The listing builds one solid part. Answer for the finished solid, in the listing's coordinates (mm). A direction names the side the tool comes from. Coordinates: 2 decimals unless noted, no trailing zeros. Order: outer loops, then holes, each group sorted by start corner. A loop starts at its lowest first (then second) coordinate and runs counter-clockwise, first axis right, second up. Notation, with made-up numbers: (-38.5, 4) -> (-15.5, 4) arc R25 cw to (-15.5, 34) -> close; hole circle Ø11 at (11.25, 79). An arc over 180 degrees is marked (long way). Answer in a Markdown table with one row per item.
```python
from build123d import *

# Parameters (mm, degrees)
BOSS_EXTRUDE1_DEPTH     = 37.5
SHELL1_T                = -10
SKETCH2_W               = 230
SKETCH2_H               = 15
BOSS_EXTRUDE3_DEPTH     = 75
SKETCH1_4_OUTSIDE_W     = 306.9
SKETCH1_4_OUTSIDE_H     = 141.9
CUT_EXTRUDE2_DEPTH      = 38.5
CUT_EXTRUDE2_DEPTH_BACK = 38.5
SKETCH4_W               = 10
SKETCH4_H               = 75
SKETCH4_R               = 2.5
BOSS_EXTRUDE4_DEPTH     = 5
FILLET1_R               = 10
SKETCH3_R               = 3.75
CUT_EXTRUDE3_DEPTH      = 35
CUT_EXTRUDE4_START      = -75
SKETCH3_13_R            = 15
CUT_EXTRUDE4_DEPTH      = 35
CUT_EXTRUDE5_START      = -5
CUT_EXTRUDE5_DEPTH      = 65
CUT_EXTRUDE6_START      = -5
CUT_EXTRUDE6_DEPTH      = 30


with BuildPart() as part:
    # Sketch1 → Boss-Extrude1 (new body, symmetric)
    with BuildSketch(Plane.XY):
        with BuildLine():
            Line((125, 0), (-125, 0))
            Line((-125, 0), (-125, -15))
            ThreePointArc((-125, -15), (-104.497474683, -64.497474683), (-55, -85))
            Line((-55, -85), (45, -85))
            ThreePointArc((45, -85), (101.568542495, -61.568542495), (125, -5))
            Line((125, -5), (125, 0))
        make_face()
    extrude(amount=BOSS_EXTRUDE1_DEPTH, both=True)

    # Shell1
    shell1_openings = [part.faces().sort_by_distance(p)[0] for p in [
        (0, 0, 0),
    ]]
    offset(amount=SHELL1_T, openings=shell1_openings, kind=Kind.INTERSECTION)

    # Sketch2 → Boss-Extrude3 (add)
    with BuildSketch(Plane(origin=(0, 0, 0), x_dir=(1, 0, 0), z_dir=(0, 1, 0))):
        Rectangle(SKETCH2_W, SKETCH2_H)
    extrude(amount=-BOSS_EXTRUDE3_DEPTH)

    # Sketch1<4> outside → Cut-Extrude2 (cut, two sides)
    with BuildSketch(Plane.XY) as cut_extrude2_sk:
        with Locations((0, -42.5)):
            Rectangle(SKETCH1_4_OUTSIDE_W, SKETCH1_4_OUTSIDE_H)
        with BuildLine():
            Line((125, 0), (-125, 0))
            Line((-125, 0), (-125, -15))
            ThreePointArc((-125, -15), (-104.497474683, -64.497474683), (-55, -85))
            Line((-55, -85), (45, -85))
            ThreePointArc((45, -85), (101.568542495, -61.568542495), (125, -5))
            Line((125, -5), (125, 0))
        make_face(mode=Mode.SUBTRACT)
    extrude(amount=CUT_EXTRUDE2_DEPTH, mode=Mode.SUBTRACT)
    extrude(cut_extrude2_sk.sketch, amount=-CUT_EXTRUDE2_DEPTH_BACK, mode=Mode.SUBTRACT)

    # Sketch4 → Boss-Extrude4 (add)
    with BuildSketch(Plane(origin=(0, 0, 0), x_dir=(1, 0, 0), z_dir=(0, 1, 0))):
        with Locations((-130, 0)):
            Rectangle(SKETCH4_W, SKETCH4_H)
        with Locations((-129.5, -30.5)):
            Circle(SKETCH4_R, mode=Mode.SUBTRACT)
        with Locations((-129.5, 30.5)):
            Circle(SKETCH4_R, mode=Mode.SUBTRACT)
        with Locations((130, 0)):
            Rectangle(SKETCH4_W, SKETCH4_H)
        with Locations((129.5, 30.5)):
            Circle(SKETCH4_R, mode=Mode.SUBTRACT)
        with Locations((129.5, -30.5)):
            Circle(SKETCH4_R, mode=Mode.SUBTRACT)
    extrude(amount=-BOSS_EXTRUDE4_DEPTH)

    # Fillet1
    fillet1_edges = [part.edges().sort_by_distance(p)[0] for p in [
        (-125, -10, -37.5),
        (-125, -10, 37.5),
        (-5, -85, 37.5),
        (-104.497474683, -64.497474683, 37.5),
        (-104.497474683, -64.497474683, -37.5),
        (-5, -85, -37.5),
        (101.568542495, -61.568542495, -37.5),
        (101.568542495, -61.568542495, 37.5),
    ]]
    fillet(fillet1_edges, radius=FILLET1_R)

    # Sketch3 → Cut-Extrude3 (cut)
    with BuildSketch(Plane(origin=(0, 0, -37.5), x_dir=(-1, 0, 0), z_dir=(0, 0, -1))):
        with Locations((54, 0)):
            Circle(SKETCH3_R)
    extrude(amount=-CUT_EXTRUDE3_DEPTH, mode=Mode.SUBTRACT)

    # Sketch3<13> → Cut-Extrude4 (cut)
    with BuildSketch(Plane(origin=(0, 0, -37.5), x_dir=(-1, 0, 0), z_dir=(0, 0, -1)).offset(CUT_EXTRUDE4_START)):
        with Locations((30, 0)):
            Circle(SKETCH3_13_R)
    extrude(amount=CUT_EXTRUDE4_DEPTH, mode=Mode.SUBTRACT)

    # Sketch3<14> → Cut-Extrude5 (cut)
    with BuildSketch(Plane(origin=(0, 0, -37.5), x_dir=(-1, 0, 0), z_dir=(0, 0, -1)).offset(CUT_EXTRUDE5_START)):
        with BuildLine():
            Line((-59, 0), (-49, 0))
            ThreePointArc((-49, 0), (-54, 5), (-59, 0))
        make_face()
        with BuildLine():
            ThreePointArc((-59, 0), (-54, -5), (-49, 0))
            Line((-49, 0), (-59, 0))
        make_face()
    extrude(amount=-CUT_EXTRUDE5_DEPTH, mode=Mode.SUBTRACT)

    # Sketch3<15> → Cut-Extrude6 (cut)
    with BuildSketch(Plane(origin=(0, 0, -37.5), x_dir=(-1, 0, 0), z_dir=(0, 0, -1)).offset(CUT_EXTRUDE6_START)):
        with BuildLine():
            Line((15, 0), (23, 0))
            ThreePointArc((23, 0), (20.581988897, 4.281744193), (15.666666667, 4.422166387))
            ThreePointArc((15.666666667, 4.422166387), (15.167603026, 2.236067977), (15, 0))
        make_face()
        with BuildLine():
            ThreePointArc((15.666666667, -4.422166387), (20.581988897, -4.281744193), (23, 0))
            Line((23, 0), (15, 0))
            ThreePointArc((15, 0), (15.167603026, -2.236067977), (15.666666667, -4.422166387))
        make_face()
        with BuildLine():
            ThreePointArc((15, 0), (15.167603026, 2.236067977), (15.666666667, 4.422166387))
            ThreePointArc((15.666666667, 4.422166387), (13.718255807, 2.581988897), (13, 0))
            Line((13, 0), (15, 0))
        make_face()
        with BuildLine():
            ThreePointArc((13, 0), (13.718255807, -2.581988897), (15.666666667, -4.422166387))
            ThreePointArc((15.666666667, -4.422166387), (15.167603026, -2.236067977), (15, 0))
            Line((15, 0), (13, 0))
        make_face()
    extrude(amount=-CUT_EXTRUDE6_DEPTH, mode=Mode.SUBTRACT)


solid = part.part
```
(1) For a pull along Z with two mould halves and no side action, classify faces 4 (the cylindrical face through (-4.3, -82.15, -34.49)), 5 (the flat face through (-130, -5, -1)), 6 (the cylindrical face through (-4.3, -82.15, 34.49)), 7 (the cylindrical face through (54, -5, -30)) as released by +Z, released by -Z, zero draft, split by the parting line, or undercut.
Check values:
| item | result |
|---|---|
| face 4 | released by -Z |
| face 5 | zero draft |
| face 6 | released by +Z |
| face 7 | undercut |
(2) A cutting plane is placed at D-D, the plane y = -62.5. Count the separate pieces of the cut face and the enclosed holes in it, then the cut area to 3 significant figures.
Check values:
| item | result |
|---|---|
| separate pieces | 1 |
| enclosed holes | 2 |
| area | 8,340 mm² |
(3) A cutting plane is placed at B-B, the plane z = 0. Determine the outline of the cut face in (x, y), then the cut area to 3 significant figures.
Check values:
| item | result |
|---|---|
| outline | (-135, -5) -> (-125, -5) -> (-125, -15) arc R70 ccw to (-55, -85) -> (45, -85) arc R80 ccw to (125, -5) -> (135, -5) -> (135, 0) -> (59, 0) arc R5 cw to (49, 0) -> (-135, 0) -> close |
| area | 18,900 mm² |
(4) Which of the six approach directions +Z, -Z, +X, -X, +Y, -Y give full straight-line access (tool end or side, diameter ignored) to faces 1 (the cylindrical face through (-30, -15, 5)), 2 (the cylindrical face through (93.95, -55.04, -17.36)), 3 (the flat face through (-125, -10, 0))?
Check values:
| item | result |
|---|---|
| face 1 | +Z, +Y |
| face 2 | +Y |
| face 3 | +Z, -Z, -X, -Y |
(5) A cutting plane is placed at C-C, the plane x = -30. Determine the outline of the cut face in (y, z), then the cut area to 3 significant figures.
Check values:
| item | result |
|---|---|
| outline | (-85, -27.5) arc R10 ccw to (-75, -37.5) -> (0, -37.5) -> (0, -27.5) -> (-75, -27.5) -> (-75, -7.5) -> (0, -7.5) -> (0, 2.5) -> (-15, 2.5) -> (-15, 7.5) -> (-75, 7.5) -> (-75, 27.5) -> (-15, 27.5) -> (-15, 37.5) -> (-75, 37.5) arc R10 ccw to (-85, 27.5) -> close |
| area | 3,110 mm² |
(6) Find the intervals of material crossed by line 1 along Z through (x, y) = (129.5, -1.95); line 2 along Z through (x, y) = (-2.5, -47.5); line 3 along X through (y, z) = (-2, 30), in increasing order. Write a range as from..to.
Check values:
| item | result |
|---|---|
| line 1 | -37.5..-33, -28..28, 33..37.5 |
| line 2 | -37.5..-27.5, -7.5..7.5, 27.5..37.5 |
| line 3 | -135..-131.95, -127.05..-44.87, -15.13..49.42, 58.58..127.05, 131.95..135 |
(7) Flat-ended cylindrical pins translate along their axes: pin 1 (22 mm diameter, centred on x = -129.5, z = -10, fed in from -Y); pin 2 (5 mm diameter, centred on y = -31.5, z = 19, fed in from -X); pin 3 (2 mm diameter, centred on x = -96.5, z = -12, fed in from -Y). Find the tip coordinate at first contact, or state that the pin passes through.
Check values:
| item | result |
|---|---|
| pin 1 | y = -44.46 |
| pin 2 | x = -123.59 |
| pin 3 | y = -72.09 |
(8) A cutting plane is placed at A-A, the plane x = -129.5. Determine the outline of the cut face in (y, z).
Check values:
| item | result |
|---|---|
| outline | (-5, -37.5) -> (0, -37.5) -> (0, -33) -> (-5, -33) -> close; (-5, -28) -> (0, -28) -> (0, 28) -> (-5, 28) -> close; (-5, 33) -> (0, 33) -> (0, 37.5) -> (-5, 37.5) -> close |
